Design review of the part built by this model. Coordinates are the model's own, in mm. A direction names the side the tool comes from. Give positions to 0.01 mm unless a question says otherwise; leave off trailing zeros. Loops run counter-clockwise (first coordinate to the right, second up) from the corner with the lowest first, then second, coordinate; pieces in that order, holes last. Notation, with made-up numbers: (74, -39) -> (120, -39) arc R7 cw to (120, -35) -> close; hole circle Ø4 at (12.5, -31.5). An arc over 180 degrees is marked (long way). Answer in a Markdown table with one row per item. Add a question column.
(1) Consider section B-B on y = 46. Write out the cut boundary in (x, z), then the cut area to 3 significant figures.
(2) For line 1 (Y direction, x = 31.5, z = 13.25); line 2 (X direction, y = -15.5, z = 1.75); line 3 (X direction, y = 9, z = 3), list the stretches that pass through material, from the lowest coordinate up.
(3) Consider section D-D on x = 40.5. Write out the cut boundary in (y, z), then the cut area to 3 significant figures.
(4) For faces 3 (the flat face through (33, -22.366, 8)), 4 (the flat face through (92, 60, 3)), 5 (the flat face through (-31, 41, 12)), 6 (the flat face through (92, -11.366, 6)), 7 (the flat face through (77.335, -21, 10)), list the 3-axis set-ups (+Z, -Z, +X, -X, +Y, -Y) from which the entire face can be reached by the end or side of a thin tool; tool diameter is ignored.
(5) Consider section C-C on z = 8.75. Write out the cut boundary in (x, y).
(6) Draft analysis for pull direction X (two halves, no side actions). For faces 1 (the flat face through (-29.465, 23, 9)), 2 (the flat face through (28, -20, 18)), state which applies: +X half, -X half, draft (parallel to the pull), parting line (faces both ways), or undercut.
(7) Consider section A-A on x = 71.5. Write out the cut boundary in (y, z), then the cut area to 3 significant figures.
from build123d import *

# Parameters (mm, degrees)
BOSS_EXTRU_1_DEPTH       = 18
BOSS_EXTRU_1_DEPTH_BACK  = 2
ESQUISSE1_W              = 132
ESQUISSE1_H              = 92
ENL_V_START              = -3
ESQUISSE14_W             = 126
ESQUISSE14_H             = 86
ENL_V_MAT_EXTRU_1_DEPTH  = 121.109755351
ESQUISSE15_W             = 8
ESQUISSE15_H             = 10
BOSS_EXTRU_2_DEPTH       = 8
ESQUISSE16_W             = 8
ESQUISSE16_H             = 10
BOSS_EXTRU_3_DEPTH       = 8
ESQUISSE17_W             = 8
ESQUISSE17_H             = 10
BOSS_EXTRU_4_DEPTH       = 8
ESQUISSE18_W             = 8
ESQUISSE18_H             = 10
BOSS_EXTRU_5_DEPTH       = 8
ESQUISSE19_R             = 1.15
ENL_V_MAT_EXTRU_2_DEPTH  = 10
ESQUISSE20_R             = 1.15
ENL_V_MAT_EXTRU_3_DEPTH  = 10
ESQUISSE21_R             = 1.15
ENL_V_MAT_EXTRU_4_DEPTH  = 10
ESQUISSE22_R             = 1.15
ENL_V_MAT_EXTRU_5_DEPTH  = 10
ENL_V_START_2            = -8
ENL_V_MAT_EXTRU_6_DEPTH  = 2
ESQUISSE24_W             = 4.34
ESQUISSE24_H             = 2
ENL_V_MAT_EXTRU_7_DEPTH  = 3
ENL_V_MAT_EXTRU_8_DEPTH  = 2
ESQUISSE26_W             = 4.34
ESQUISSE26_H             = 2
ENL_V_MAT_EXTRU_9_DEPTH  = 3
ENL_V_MAT_EXTRU_10_DEPTH = 2
ESQUISSE28_W             = 4.34
ESQUISSE28_H             = 2
ENL_V_MAT_EXTRU_11_DEPTH = 3
ENL_V_MAT_EXTRU_12_DEPTH = 2
ESQUISSE30_W             = 4.34
ESQUISSE30_H             = 2
ENL_V_MAT_EXTRU_13_DEPTH = 3
ESQUISSE31_W             = 10
ESQUISSE31_H             = 6
ENL_V_MAT_EXTRU_14_DEPTH = 3
ESQUISSE32_W             = 2.85
ESQUISSE32_H             = 15
ENL_V_MAT_EXTRU_15_DEPTH = 3
CONG_1_R                 = 0.5
CONG_2_R                 = 0.5
CONG_3_R                 = 0.5
CONG_4_R                 = 0.5


with BuildPart() as part:
    # Esquisse1 → Boss.-Extru.1 (new, two sides: drawn at the far end of the back side and taken through both)
    with BuildSketch(Plane.XY.offset(-BOSS_EXTRU_1_DEPTH_BACK)):
        with Locations((33.534709402, 23.633709415)):
            Rectangle(ESQUISSE1_W, ESQUISSE1_H)
    extrude(amount=BOSS_EXTRU_1_DEPTH + BOSS_EXTRU_1_DEPTH_BACK)

    # Esquisse14 → Enlèv. mat.-Extru.1 (cut, through all)
    with BuildSketch(Plane(origin=(0, 0, -2), x_dir=(-1, 0, 0), z_dir=(0, 0, -1)).offset(ENL_V_START)):
        with Locations((-33.534709402, 23.633709415)):
            Rectangle(ESQUISSE14_W, ESQUISSE14_H)
    extrude(amount=-ENL_V_MAT_EXTRU_1_DEPTH, mode=Mode.SUBTRACT)

    # Esquisse15 → Boss.-Extru.2 (add)
    with BuildSketch(Plane(origin=(0, 66.633709415, 0), x_dir=(-1, 0, 0), z_dir=(0, -1, 0))):
        with Locations((25.465290598, -6)):
            Rectangle(ESQUISSE15_W, ESQUISSE15_H)
    extrude(amount=BOSS_EXTRU_2_DEPTH)

    # Esquisse16 → Boss.-Extru.3 (add)
    with BuildSketch(Plane(origin=(0, 66.633709415, 0), x_dir=(-1, 0, 0), z_dir=(0, -1, 0))):
        with Locations((-92.534709402, -6)):
            Rectangle(ESQUISSE16_W, ESQUISSE16_H)
    extrude(amount=BOSS_EXTRU_3_DEPTH)

    # Esquisse17 → Boss.-Extru.4 (add)
    with BuildSketch(Plane(origin=(0, -19.366290585, 0), x_dir=(1, 0, 0), z_dir=(0, 1, 0))):
        with Locations((92.534709402, -6)):
            Rectangle(ESQUISSE17_W, ESQUISSE17_H)
    extrude(amount=BOSS_EXTRU_4_DEPTH)

    # Esquisse18 → Boss.-Extru.5 (add)
    with BuildSketch(Plane(origin=(0, -19.366290585, 0), x_dir=(1, 0, 0), z_dir=(0, 1, 0))):
        with Locations((-25.465290598, -6)):
            Rectangle(ESQUISSE18_W, ESQUISSE18_H)
    extrude(amount=BOSS_EXTRU_5_DEPTH)

    # Esquisse19 → Enlèv. mat.-Extru.2 (cut)
    with BuildSketch(Plane.XY.offset(11)):
        with Locations((92.034709402, -15.366290585)):
            Circle(ESQUISSE19_R)
    extrude(amount=-ENL_V_MAT_EXTRU_2_DEPTH, mode=Mode.SUBTRACT)

    # Esquisse20 → Enlèv. mat.-Extru.3 (cut)
    with BuildSketch(Plane.XY.offset(11)):
        with Locations((-24.965290598, -15.366290585)):
            Circle(ESQUISSE20_R)
    extrude(amount=-ENL_V_MAT_EXTRU_3_DEPTH, mode=Mode.SUBTRACT)

    # Esquisse21 → Enlèv. mat.-Extru.4 (cut)
    with BuildSketch(Plane.XY.offset(11)):
        with Locations((-24.965290598, 61.633709415)):
            Circle(ESQUISSE21_R)
    extrude(amount=-ENL_V_MAT_EXTRU_4_DEPTH, mode=Mode.SUBTRACT)

    # Esquisse22 → Enlèv. mat.-Extru.5 (cut)
    with BuildSketch(Plane.XY.offset(11)):
        with Locations((92.034709402, 61.633709415)):
            Circle(ESQUISSE22_R)
    extrude(amount=-ENL_V_MAT_EXTRU_5_DEPTH, mode=Mode.SUBTRACT)

    # Esquisse23 → Enlèv. mat.-Extru.6 (cut)
    with BuildSketch(Plane.XY.offset(11).offset(ENL_V_START_2)):
        Polygon((89.869645893, -14.116290585), (89.869645893, -16.616290585), (92.034709402, -17.866290585), (94.199772912, -16.616290585), (94.199772912, -14.116290585), (92.034709402, -12.866290585), align=None)
    extrude(amount=-ENL_V_MAT_EXTRU_6_DEPTH, mode=Mode.SUBTRACT)

    # Esquisse24 → Enlèv. mat.-Extru.7 (cut)
    with BuildSketch(Plane(origin=(0, -11.366290585, 0), x_dir=(1, 0, 0), z_dir=(0, 1, 0))):
        with Locations((92.034709402, -2)):
            Rectangle(ESQUISSE24_W, ESQUISSE24_H)
    extrude(amount=-ENL_V_MAT_EXTRU_7_DEPTH, mode=Mode.SUBTRACT)

    # Esquisse25 → Enlèv. mat.-Extru.8 (cut)
    with BuildSketch(Plane.XY.offset(11).offset(ENL_V_START_2)):
        Polygon((-22.800227088, -14.116290585), (-24.965290598, -12.866290585), (-27.130354107, -14.116290585), (-27.130354107, -16.616290585), (-24.965290598, -17.866290585), (-22.800227088, -16.616290585), align=None)
    extrude(amount=-ENL_V_MAT_EXTRU_8_DEPTH, mode=Mode.SUBTRACT)

    # Esquisse26 → Enlèv. mat.-Extru.9 (cut)
    with BuildSketch(Plane(origin=(0, -11.366290585, 0), x_dir=(1, 0, 0), z_dir=(0, 1, 0))):
        with Locations((-24.965290598, -2)):
            Rectangle(ESQUISSE26_W, ESQUISSE26_H)
    extrude(amount=-ENL_V_MAT_EXTRU_9_DEPTH, mode=Mode.SUBTRACT)

    # Esquisse27 → Enlèv. mat.-Extru.10 (cut)
    with BuildSketch(Plane.XY.offset(11).offset(ENL_V_START_2)):
        Polygon((-24.965290598, 59.133709415), (-22.800227088, 60.383709415), (-22.800227088, 62.883709415), (-24.965290598, 64.133709415), (-27.130354107, 62.883709415), (-27.130354107, 60.383709415), align=None)
    extrude(amount=-ENL_V_MAT_EXTRU_10_DEPTH, mode=Mode.SUBTRACT)

    # Esquisse28 → Enlèv. mat.-Extru.11 (cut)
    with BuildSketch(Plane(origin=(0, 58.633709415, 0), x_dir=(-1, 0, 0), z_dir=(0, -1, 0))):
        with Locations((24.965290598, -2)):
            Rectangle(ESQUISSE28_W, ESQUISSE28_H)
    extrude(amount=-ENL_V_MAT_EXTRU_11_DEPTH, mode=Mode.SUBTRACT)

    # Esquisse29 → Enlèv. mat.-Extru.12 (cut)
    with BuildSketch(Plane.XY.offset(11).offset(ENL_V_START_2)):
        Polygon((89.869645893, 60.383709415), (92.034709402, 59.133709415), (94.199772912, 60.383709415), (94.199772912, 62.883709415), (92.034709402, 64.133709415), (89.869645893, 62.883709415), align=None)
    extrude(amount=-ENL_V_MAT_EXTRU_12_DEPTH, mode=Mode.SUBTRACT)

    # Esquisse30 → Enlèv. mat.-Extru.13 (cut)
    with BuildSketch(Plane(origin=(0, 58.633709415, 0), x_dir=(-1, 0, 0), z_dir=(0, -1, 0))):
        with Locations((-92.034709402, -2)):
            Rectangle(ESQUISSE30_W, ESQUISSE30_H)
    extrude(amount=-ENL_V_MAT_EXTRU_13_DEPTH, mode=Mode.SUBTRACT)

    # Esquisse31 → Enlèv. mat.-Extru.14 (cut)
    with BuildSketch(Plane(origin=(0, -19.366290585, 0), x_dir=(1, 0, 0), z_dir=(0, 1, 0))):
        with Locations((72.334709402, -9.8)):
            Rectangle(ESQUISSE31_W, ESQUISSE31_H)
    extrude(amount=-ENL_V_MAT_EXTRU_14_DEPTH, mode=Mode.SUBTRACT)

    # Esquisse32 → Enlèv. mat.-Extru.15 (cut)
    with BuildSketch(Plane(origin=(-29.465290598, 0, 0), x_dir=(0, 0, -1), z_dir=(1, 0, 0))):
        with Locations((-13.425, 41.203709415)):
            Rectangle(ESQUISSE32_W, ESQUISSE32_H)
    extrude(amount=-ENL_V_MAT_EXTRU_15_DEPTH, mode=Mode.SUBTRACT)

    # Congé1
    cong_1_edges = [part.edges().sort_by_distance(p)[0] for p in [
        (-32.465290598, 69.633709415, 8),
    ]]
    fillet(cong_1_edges, radius=CONG_1_R)

    # Congé2
    cong_2_edges = [part.edges().sort_by_distance(p)[0] for p in [
        (-32.465290598, -22.366290585, 8),
    ]]
    fillet(cong_2_edges, radius=CONG_2_R)

    # Congé3
    cong_3_edges = [part.edges().sort_by_distance(p)[0] for p in [
        (99.534709402, -22.366290585, 8),
    ]]
    fillet(cong_3_edges, radius=CONG_3_R)

    # Congé4
    cong_4_edges = [part.edges().sort_by_distance(p)[0] for p in [
        (99.534709402, 69.633709415, 8),
    ]]
    fillet(cong_4_edges, radius=CONG_4_R)


solid = part.part
Values follow:
| question | item | result |
|---|---|---|
| 1 | outline | (-32.47, -2) -> (99.53, -2) -> (99.53, 18) -> (96.53, 18) -> (96.53, 1) -> (-29.47, 1) -> (-29.47, 12) -> (-32.47, 12) -> close; (-32.47, 14.85) -> (-29.47, 14.85) -> (-29.47, 18) -> (-32.47, 18) -> close |
| 1 | area | 489 mm2 |
| 2 | line 1 | -22.37 to -19.37, 66.63 to 69.63 |
| 2 | line 2 | -32.47 to -27.13, -22.8 to -21.47, 88.53 to 89.87, 94.2 to 99.53 |
| 2 | line 3 | -32.47 to -29.47, 96.53 to 99.53 |
| 3 | outline | (-22.37, -2) -> (69.63, -2) -> (69.63, 18) -> (66.63, 18) -> (66.63, 1) -> (-19.37, 1) -> (-19.37, 18) -> (-22.37, 18) -> close |
| 3 | area | 378 mm2 |
| 4 | face 3 | +Z, -Z, +X, -X, -Y |
| 4 | face 4 | none |
| 4 | face 5 | -X |
| 4 | face 6 | +Z |
| 4 | face 7 | -Y |
| 5 | outline | (-32.47, -21.87) arc R0.5 ccw to (-31.97, -22.37) -> (67.33, -22.37) -> (67.33, -19.37) -> (-21.47, -19.37) -> (-21.47, -11.37) -> (-29.47, -11.37) -> (-29.47, 58.63) -> (-21.47, 58.63) -> (-21.47, 66.63) -> (88.53, 66.63) -> (88.53, 58.63) -> (96.53, 58.63) -> (96.53, -11.37) -> (88.53, -11.37) -> (88.53, -19.37) -> (77.33, -19.37) -> (77.33, -22.37) -> (99.03, -22.37) arc R0.5 ccw to (99.53, -21.87) -> (99.53, 69.13) arc R0.5 ccw to (99.03, 69.63) -> (-31.97, 69.63) arc R0.5 ccw to (-32.47, 69.13) -> close; hole circle Ø2.3 at (-24.97, -15.37); hole circle Ø2.3 at (-24.97, 61.63); hole circle Ø2.3 at (92.03, -15.37); hole circle Ø2.3 at (92.03, 61.63) |
| 6 | face 1 | undercut |
| 6 | face 2 | draft |
| 7 | outline | (-22.37, -2) -> (69.63, -2) -> (69.63, 18) -> (66.63, 18) -> (66.63, 1) -> (-19.37, 1) -> (-19.37, 6.8) -> (-22.37, 6.8) -> close; (-22.37, 12.8) -> (-19.37, 12.8) -> (-19.37, 18) -> (-22.37, 18) -> close |
| 7 | area | 360 mm2 |
